from build123d import *

# Parameters (mm, degrees)
F0_W           = 128.5
F0_H           = 102
F1_DEPTH       = 5
F3_DEPTH       = 5
F5_D           = 5
F8_D           = 3.5
F8_CBORE_D     = 6
F8_CBORE_DEPTH = 2.5


with BuildPart() as f1:
    # F0 (on Top) → F1 (new body)
    with BuildSketch(Plane.XY):
        Rectangle(F0_W, F0_H)
    extrude(amount=F1_DEPTH)

    # F2 (on face) → F3 (join)
    with BuildSketch(Plane.XZ.offset(51)):
        with BuildLine():
            Line((-64.25, 12.5), (-64.25, 5))
            Line((-64.25, 5), (-54.25, 5))
            Line((-54.25, 5), (-54.25, 12.5))
            ThreePointArc((-54.25, 12.5), (-59.25, 17.5), (-64.25, 12.5))
        make_face()
        with BuildLine():
            Line((54.25, 12.5), (54.25, 5))
            Line((54.25, 5), (64.25, 5))
            Line((64.25, 5), (64.25, 12.5))
            ThreePointArc((64.25, 12.5), (59.25, 17.5), (54.25, 12.5))
        make_face()
    extrude(amount=-F3_DEPTH)

    # F5 (through all)
    with Locations(Plane.XZ.offset(51)):
        with Locations((-59.25, 12.5), (59.25, 12.5)):
            Hole(F5_D / 2)

    # F6: F1 across plane


with BuildPart() as f1_1:
    add(f1.part)
    add(f1.part.mirror(Plane.XZ))

    # F8 (through all)
    with Locations(Plane.XY.offset(5)):
        with Locations((-37, 18.5), (-37, -18.5), (37, 0)):
            CounterBoreHole(F8_D / 2, F8_CBORE_D / 2, F8_CBORE_DEPTH)


solid = f1_1.part
The model under review builds one solid part; all positions refer to its coordinate system, in mm. A direction names the side the tool comes from. Coordinates: 2 decimals unless noted, no trailing zeros. Write each loop counter-clockwise with the first axis right and the second up, starting at its lowest first coordinate (ties: lowest second). Pieces come first, ordered by that corner, then holes. Notation, with made-up numbers: (63, -27) - (77, -27) arc R18 cw to (77, -8) - close; hole circle Ø11 at (61.5, -39.5). An arc over 180 degrees is marked (long way). Answer as a JSON object with one key per item and string values. Group by question number.
1. To check wall thickness, follow probe 1 along Y at (x, z) = (-37, 1.8); probe 2 along Y at (x, z) = (-37, 4.5); probe 3 along Z at (x, y) = (59.25, 48.55). State the ranges of each line that lie inside material, in increasing order.
2. Mouldability with a two-part tool opening along Y and no side actions: class faces 1 (the face through (-1, 51, 3)), 2 (the face through (-37, 16.5, 2.5)), 3 (the face through (-60.4, -46, 9.9)), 4 (the face through (-1, 1, 0)) as pulls with the +Y half, pulls with the -Y half, needs draft (parallel to the pull), parting line crosses it, or undercut.
3. Add section B-B (y = -18.5). Give the boundary of the cut face in (x, z), plus the area to 3 significant figures.
4. Machinability: for faces 5 (the face through (59.36, -48.54, 17.5)), 6 (the face through (58, 46, 10)), 7 (the face through (39, 0, 2.5)), which of the approach directions +Z, -Z, +X, -X, +Y, -Y give a long, thin tool a straight path to every point of the face, cutting with its end or side? Answer none if there is none.
5. Add section A-A (x = -37). Give the boundary of the cut face in (y, z), plus the area to 4 significant figures.
6. Clearance check with flat-ended pins moving along their axes: pin 1 Ø6.5 at (x, y) = (36.5, 1.5) entering from +Z; pin 2 Ø1.8 at (x, y) = (-37.5, 20) entering from +Z. State where each tip first meets the part, or that it passes through.
7. Add section D-D (x = -59.25). Give the boundary of the cut face in (y, z), plus the area to 3 significant figures.
8. Add section C-C (x = 37). Give the boundary of the cut face in (y, z).
Findings:
{
 "1": {"probe 1": "-51 to -20.25, -16.75 to 16.75, 20.25 to 51", "probe 2": "-51 to -21.5, -15.5 to 15.5, 21.5 to 51", "probe 3": "0 to 10, 15 to 17.5"},
 "2": {"face 1": "pulls with the +Y half", "face 2": "undercut", "face 3": "undercut", "face 4": "needs draft"},
 "3": {"outline": "(-64.25, 0) - (-38.75, 0) - (-38.75, 2.5) - (-40, 2.5) - (-40, 5) - (-64.25, 5) - close; (-35.25, 0) - (64.25, 0) - (64.25, 5) - (-34, 5) - (-34, 2.5) - (-35.25, 2.5) - close", "area": "619 mm²"},
 "4": {"face 5": "+Z, +Y, -Y", "face 6": "+Z, +X, -X", "face 7": "+Z"},
 "5": {"outline": "(-51, 0) - (-20.25, 0) - (-20.25, 2.5) - (-21.5, 2.5) - (-21.5, 5) - (-51, 5) - close; (-16.75, 0) - (16.75, 0) - (16.75, 2.5) - (15.5, 2.5) - (15.5, 5) - (-15.5, 5) - (-15.5, 2.5) - (-16.75, 2.5) - close; (20.25, 0) - (51, 0) - (51, 5) - (21.5, 5) - (21.5, 2.5) - (20.25, 2.5) - close", "area": "462.5 mm²"},
 "6": {"pin 1": "z = 5", "pin 2": "z = 2.5"},
 "7": {"outline": "(-51, 0) - (51, 0) - (51, 10) - (46, 10) - (46, 5) - (-46, 5) - (-46, 10) - (-51, 10) - close; (-51, 15) - (-46, 15) - (-46, 17.5) - (-51, 17.5) - close; (46, 15) - (51, 15) - (51, 17.5) - (46, 17.5) - close", "area": "585 mm²"},
 "8": {"outline": "(-51, 0) - (-1.75, 0) - (-1.75, 2.5) - (-3, 2.5) - (-3, 5) - (-51, 5) - close; (1.75, 0) - (51, 0) - (51, 5) - (3, 5) - (3, 2.5) - (1.75, 2.5) - close"}
}
